The model under review builds one solid part; all positions refer to its coordinate system, in mm. Face numbers are marked on the shaded views. A direction names the side the tool comes from. Round coordinates to 2 decimals unless told otherwise and drop trailing zeros. Write each loop counter-clockwise with the first axis right and the second up, starting at its lowest first coordinate (ties: lowest second). Pieces come first, ordered by that corner, then holes. Notation, with made-up numbers: (37.25, 22) - (87.25, 22) arc R22 cw to (87.25, 39) - close; hole circle Ø1 at (73.25, -13). An arc over 180 degrees is marked (long way). Return JSON: item names as keys, results as strings.
Autodesk Inventor part; units mm, degrees
ref_plane "XZ Plane" through (0, 0, 0) normal (0, 1, 0) x (-1, 0, 0)
ref_plane "XY Plane" through (0, 0, 0) normal (0, 0, 1) x (1, 0, 0)
sketch "Sketch1" plane through (0, 0, 0) normal (0, 1, 0) x (-1, 0, 0)
  circle A0 centre (0, 0) radius 7.5
  circle A1 centre (0, 0) radius 2.75
  dimension "d0" = 15
  dimension "d1" = 5.5
extrude "Extrusion1" add sketch "Sketch1" along normal blind 14
sketch "Sketch2" plane through (0, 14, 0) normal (0, 1, 0) x (1, 0, 0)
  circle A0 centre (0, 0) radius 2.75
  circle A1 centre (0, 0) radius 2.75
  circle A2 centre (0, 0) radius 4
  dimension "d4" = 5.5
  dimension "d5" = 8
extrude "Extrusion2" add sketch "Sketch2" along normal blind 6
fillet "Fillet1" radius 6 1 edges at (-4, 14, 0)
fillet "Fillet2" radius 6 2 edges at (0, 14, -7.5) (0, 14, 7.5)
ref_plane "Work Plane1" through (12.5, 0, 0) normal (1, 0, 0) x (0, 1, 0)
mirror "Mirror1" about plane through (12.5, 0, 0) normal (1, 0, 0) of "Extrusion1", "Extrusion2", "Fillet1", "Fillet2"
sketch "Sketch3" plane through (0, 0, 0) normal (0, 1, 0) x (-1, 0, 0)
  circle A0 centre (-25, 0) radius 2.75
  line L0 (-25, 0) -> (-25, 2.75)
  line L1 (-25, 0) -> (-25, -2.75)
  line L2 (0, 0) -> (0, -2.75)
  circle A1 centre (0, 0) radius 2.75
  line L3 (0, 0) -> (0, 2.75)
  line L4 (-25, 2.75) -> (0, 2.75)
  line L5 (0, 2.75) -> (0, 7.5)
  line L6 (0, 7.5) -> (-25, 7.5)
  line L7 (-25, 7.5) -> (-25, 2.75)
  line L8 (-25, -2.75) -> (0, -2.75)
  line L9 (0, -2.75) -> (0, -7.5)
  line L10 (0, -7.5) -> (-25, -7.5)
  line L11 (-25, -7.5) -> (-25, -2.75)
  dimension "d11" = 25
  dimension "d12" = 4.75
  dimension "d13" = 25
  dimension "d14" = 4.75
extrude "Extrusion3" add sketch "Sketch3" along normal blind 11 contours A0 L4 A1 L8 | L7 L6 L5 L4 | L8 L9 L10 L11
properties part number "4mm_Roller_Spacer_simple"
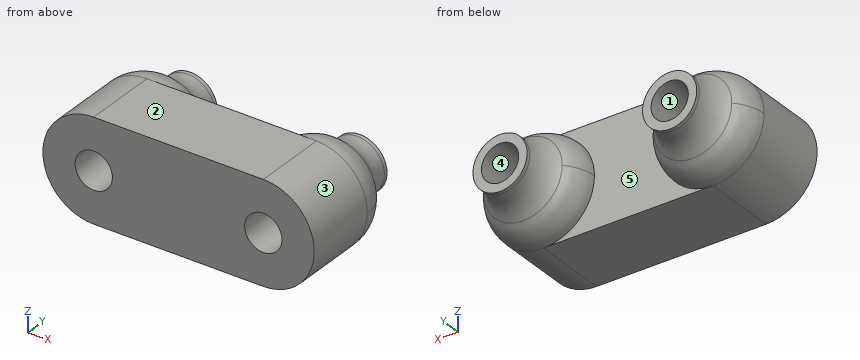
(1) Add section C-C (z = -1.5). Give the number of separate pieces and of enclosed holes in the cut face, plus the area to 3 significant figures.
Filled in:
{"separate pieces": "3", "enclosed holes": "0", "area": "448 mm2"}
(2) Clearance check with a flat-ended pin moving along its axis: pin 1 Ø3 at (x, y) = (20.5, 17.5) entering from +Z. State where the tip first meets the part, or that it passes through.
Filled in:
{"pin 1": "stops at z = 3.38"}
(3) For the marked faces 4 and 5, list the 3-axis set-ups (+Z, -Z, +X, -X, +Y, -Y) from which the entire face can be reached by the end or side of a thin tool; tool diameter is ignored.
Filled in:
{"face 4": "+Y, -Y", "face 5": "+Y"}
(4) Add section A-A (y = 4.5). Write out the cut boundary in (x, z), plus the area to 3 significant figures.
Filled in:
{"outline": "(0, -7.5) - (25, -7.5) arc R7.5 ccw to (25, 7.5) - (0, 7.5) arc R7.5 ccw to start; hole circle Ø5.5 at (0, 0); hole circle Ø5.5 at (25, 0)", "area": "504 mm2"}
(5) Mouldability with a two-part tool opening along Z and no side actions: class the marked faces 1, 2 and 3 as released by +Z, released by -Z, zero draft, split by the parting line, or undercut.
Filled in:
{"face 1": "undercut", "face 2": "released by +Z", "face 3": "split by the parting line"}
(6) Wall thickness on line 1 (X direction, y = 4.75, z = 0); line 2 (Z direction, x = 0, y = 10.25); line 3 (X direction, y = 2.25, z = -2.5): over which ranges is each line inside the solid? List them lowest first.
Filled in:
{"line 1": "x = -7.5 to -2.75, 2.75 to 22.25, 27.75 to 32.5", "line 2": "z = -7.5 to -2.75, 2.75 to 7.5", "line 3": "x = -7.07 to -1.15, 1.15 to 23.85, 26.15 to 32.07"}
(7) Add section B-B (y = 16.5). Write out the cut boundary in (x, z), plus the area to 3 significant figures.
Filled in:
{"outline": "circle Ø9.56 at (0, 0); circle Ø9.56 at (25, 0); hole circle Ø5.5 at (0, 0); hole circle Ø5.5 at (25, 0)", "area": "95.9 mm2"}
